The model under review builds one solid part; all positions refer to its coordinate system, in mm. A direction names the side the tool comes from. Coordinates: 2 decimals unless noted, no trailing zeros. Loops run counter-clockwise (first coordinate to the right, second up) from the corner with the lowest first, then second, coordinate; pieces in that order, holes last. Notation, with made-up numbers: M 11,30 L 41,30 A28 ccw 41,63 Z; hole C -18,-25.5 d5. An arc over 180 degrees is marked long. Use CSV: the item, a comma, the result in double quotes. Start each with the question number.
1. Add section D-D, the plane y = 52.5. Write out the cut boundary in (x, z), then the cut area to 3 significant figures.
2. Add section C-C, the plane x = -5. Write out the cut boundary in (y, z), then the cut area to 3 significant figures.
3. Clearance check with flat-ended pins moving along their axes: P1, Ø1.3, axis at y = 1, z = 16.5, coming from the +X side (3 decimals); P2, Ø10, axis at x = 1.5, y = 49, coming from the +Z side; P3, Ø1, axis at x = -40, z = 9, coming from the +Y side. State where each tip first meets the part, or that it passes through.
4. For L1, parallel to Y at x = -59, z = 6.5; L2, parallel to Y at x = -5.5, z = 35.5; L3, parallel to Y at x = -2, z = 58, list the stretches that pass through material, from the lowest coordinate up.
5. Tool access review of faces 4 (the flat face through (0, 3, 18.034)), 5 (the cylindrical face through (-0.178, 27.76, 25.636)), 6 (the flat face through (-11.467, 55.453, 50.815)): name each direction out of +Z, -Z, +X, -X, +Y, -Y from which nothing blocks a thin tool from reaching the whole face with its end or side.
6. Draft analysis for pull direction Z (two halves, no side actions). For faces 1 (the cylindrical face through (-0.178, 28.225, 23.053)), 2 (the flat face through (1, 3, -22.606)), 3 (the flat face through (9.144, 56, 50)), state which applies: +Z half, -Z half, draft (parallel to the pull), parting line (faces both ways), or undercut.
7. Add section B-B, the plane z = 32. Write out the cut boundary in (x, y) (3 decimals), then the cut area to 3 significant figures.
8. Add section A-A, the plane x = 27. Write out the cut boundary in (y, z).
from build123d import *

# Parameters (mm, degrees)
SKETCH1_W                = 234.95
SKETCH1_H                = 69.596
BOSS_EXTRUDE1_DEPTH      = 2.54
SKETCH2_W                = 241.3
SKETCH2_H                = 75.946
BOSS_EXTRUDE2_DEPTH      = 2.54
SKETCH3_W                = 25.4
SKETCH3_H                = 4.572
SKETCH3_H_2              = 30.48
CUT_EXTRUDE2_DEPTH       = 127.5866408
BOSS_EXTRUDE7_DEPTH      = 12.7
BOSS_EXTRUDE7_DEPTH_BACK = 12.7
SKETCH5_W                = 25.4
SKETCH5_H                = 2.54
BOSS_EXTRUDE8_DEPTH      = 30.48
CUT_EXTRUDE3_REACH       = 153.329
SKETCH6_W                = 18.288
SKETCH6_H                = 23.01875
CUT_EXTRUDE4_REACH       = 153.329
SKETCH9_R                = 1
CUT_EXTRUDE6_REACH       = 151.523


with BuildPart() as part:
    # Sketch1 → Boss-Extrude1 (new body)
    with BuildSketch(Plane(origin=(0, 0, 0), x_dir=(1, 0, 0), z_dir=(0, 1, 0))):
        Rectangle(SKETCH1_W, SKETCH1_H)
    extrude(amount=BOSS_EXTRUDE1_DEPTH)

    # Sketch2 → Boss-Extrude2 (add)
    with BuildSketch(Plane(origin=(0, 2.54, 0), x_dir=(1, 0, 0), z_dir=(0, 1, 0))):
        Rectangle(SKETCH2_W, SKETCH2_H)
    extrude(amount=BOSS_EXTRUDE2_DEPTH)

    # Sketch3 → Cut-Extrude2 (cut, through all)
    with BuildSketch(Plane(origin=(0, 5.08, 0), x_dir=(1, 0, 0), z_dir=(0, 1, 0))):
        Polygon((102.87, 22.606), (-102.87, 22.606), (-102.87, 17.018), (-12.7, 17.018), (12.7, 17.018), (102.87, 17.018), align=None)
        with Locations((0, 14.732)):
            Rectangle(SKETCH3_W, SKETCH3_H)
        with Locations((0, -2.794)):
            Rectangle(SKETCH3_W, SKETCH3_H_2)
    extrude(amount=-CUT_EXTRUDE2_DEPTH, mode=Mode.SUBTRACT)

    # Sketch4 → Boss-Extrude7 (add, two sides: drawn at the far end of the back side and taken through both)
    with BuildSketch(Plane(origin=(0, 0, 0), x_dir=(0, 0, -1), z_dir=(1, 0, 0)).offset(-BOSS_EXTRUDE7_DEPTH_BACK)):
        with BuildLine():
            Line((-20.574, 5.08), (-18.034, 5.08))
            ThreePointArc((-18.034, 5.08), (-23.194025065, 28.533326897), (-37.721134665, 47.655238095))
            Line((-37.721134665, 47.655238095), (-39.366264908, 45.72))
            ThreePointArc((-39.366264908, 45.72), (-25.499478471, 27.467266584), (-20.574, 5.08))
        make_face()
    extrude(amount=BOSS_EXTRUDE7_DEPTH + BOSS_EXTRUDE7_DEPTH_BACK)

    # Sketch5 → Boss-Extrude8 (add)
    with BuildSketch(Plane(origin=(0, 38.605953422, 45.413858329), x_dir=(1, 0, 0), z_dir=(0, 0.6476890718445453, 0.7619047619047618))):
        with Locations((0, 10.607186134)):
            Rectangle(SKETCH5_W, SKETCH5_H)
    extrude(amount=BOSS_EXTRUDE8_DEPTH)

    # Sketch6 → Cut-Extrude3 (cut, up to next)
    with BuildSketch(Plane(origin=(0, 9.049284674, -7.692723663), x_dir=(1, 0, 0), z_dir=(0, 0.7619047619047616, -0.6476890718445452)), mode=Mode.PRIVATE) as cut_extrude3_sk1:
        with Locations((0, -74.455715595)):
            Rectangle(SKETCH6_W, SKETCH6_H)
    cut_extrude3_tool1 = extrude(cut_extrude3_sk1.sketch, amount=-CUT_EXTRUDE3_REACH, mode=Mode.PRIVATE) & part.part
    add(cut_extrude3_tool1.solids().sort_by_distance((0, 57.273438, 49.035441))[0], mode=Mode.SUBTRACT)

    # Sketch9 → Cut-Extrude4 (cut, up to next)
    with BuildSketch(Plane(origin=(0, 9.049284674, -7.692723663), x_dir=(1, 0, 0), z_dir=(0, 0.7619047619047616, -0.6476890718445452)), mode=Mode.PRIVATE) as cut_extrude4_sk1:
        with Locations(Location((-10.31875, -85.171340595, 0), (0, 0, 270))):
            Circle(SKETCH9_R)
    cut_extrude4_tool1 = extrude(cut_extrude4_sk1.sketch, amount=-CUT_EXTRUDE4_REACH, mode=Mode.PRIVATE) & part.part
    # Sketch9 → Cut-Extrude4 (cut, up to next)
    with BuildSketch(Plane(origin=(0, 9.049284674, -7.692723663), x_dir=(1, 0, 0), z_dir=(0, 0.7619047619047616, -0.6476890718445452)), mode=Mode.PRIVATE) as cut_extrude4_sk2:
        with Locations(Location((10.31875, -85.171340595, 0), (0, 0, 270))):
            Circle(SKETCH9_R)
    cut_extrude4_tool2 = extrude(cut_extrude4_sk2.sketch, amount=-CUT_EXTRUDE4_REACH, mode=Mode.PRIVATE) & part.part
    add(cut_extrude4_tool1.solids().sort_by_distance((-10.31875, 64.213831, 57.199726))[0], mode=Mode.SUBTRACT)
    add(cut_extrude4_tool2.solids().sort_by_distance((10.31875, 64.213831, 57.199726))[0], mode=Mode.SUBTRACT)

    # Sketch10 → Cut-Extrude6 (cut, up to next)
    with BuildSketch(Plane(origin=(0, 5.08, 0), x_dir=(1, 0, 0), z_dir=(0, 1, 0)), mode=Mode.PRIVATE) as cut_extrude6_sk1:
        with BuildLine():
            Line((62.300670098, 6.472268969), (64.500670098, 6.472268969))
            Line((64.500670098, 6.472268969), (64.500670098, 5.272268969))
            ThreePointArc((64.500670098, 5.272268969), (63.400670098, -16.171303867), (62.300670098, 5.272268969))
            Line((62.300670098, 5.272268969), (62.300670098, 6.472268969))
        make_face()
    cut_extrude6_tool1 = extrude(cut_extrude6_sk1.sketch, amount=-CUT_EXTRUDE6_REACH, mode=Mode.PRIVATE) & part.part
    add(cut_extrude6_tool1.solids().sort_by_distance((63.40067, 5.08, 5.342182))[0], mode=Mode.SUBTRACT)


solid = part.part
Computed:
1,outline,"M -12.7,43.42 L -9.14,43.42 L -9.14,47.34 L -12.7,47.34 Z; M 9.14,43.42 L 12.7,43.42 L 12.7,47.34 L 9.14,47.34 Z"
1,area,"27.9 mm^2"
2,outline,"M 0,-34.8 L 2.54,-34.8 L 2.54,-37.97 L 5.08,-37.97 L 5.08,-22.61 L 0,-22.61 Z; M 0,18.03 L 5.08,18.03 A55.88 ccw 47.66,37.72 L 49.82,40.27 L 47.88,41.91 L 45.72,39.37 A53.34 cw 5.08,20.57 L 5.08,37.97 L 2.54,37.97 L 2.54,34.8 L 0,34.8 Z; M 62.79,59.45 L 64.73,57.8 L 67.4,60.94 L 65.46,62.59 Z"
2,area,"302 mm^2"
3,P1,"stops at x = 117.475"
3,P2,"stops at z = 41.91"
3,P3,"stops at y = 5.08"
4,L1,"y = 0 to 5.08"
4,L2,"y = 2.54 to 5.08, 42.09 to 45.66"
4,L3,"y = 64.5 to 64.89"
5,face 4,"+Y, -Y"
5,face 5,"+Z, +X, -X"
5,face 6,"+Z, +X, -X, -Y"
6,face 1,"-Z half"
6,face 2,"undercut"
6,face 3,"draft"
7,outline,"M -120.65,2.54 L -117.475,2.54 L -117.475,0 L 117.475,0 L 117.475,2.54 L 120.65,2.54 L 120.65,5.08 L -120.65,5.08 Z; M -12.7,38.07 L 12.7,38.07 L 12.7,42.037 L -12.7,42.037 Z"
7,area,"1,310 mm^2"
8,outline,"M 0,-34.8 L 2.54,-34.8 L 2.54,-37.97 L 5.08,-37.97 L 5.08,-22.61 L 0,-22.61 Z; M 0,-17.02 L 5.08,-17.02 L 5.08,37.97 L 2.54,37.97 L 2.54,34.8 L 0,34.8 Z"
